Can you work these out from the drawing? Everything is in mm from the part's minimum corner. Give positions to 0.01 mm unless a question says otherwise; leave off trailing zeros. Order: outer loops, then holes, each group sorted by start corner. A loop starts at its lowest first (then second) coordinate and runs counter-clockwise, first axis right, second up. Notation, with made-up numbers: M 2.25,45.5 L 53.25,45.5 A7 ccw 53.25,56.5 Z; hole C 26,11 d3. An arc over 180 degrees is marked long. Answer as a JSON object with one key per item and string values.
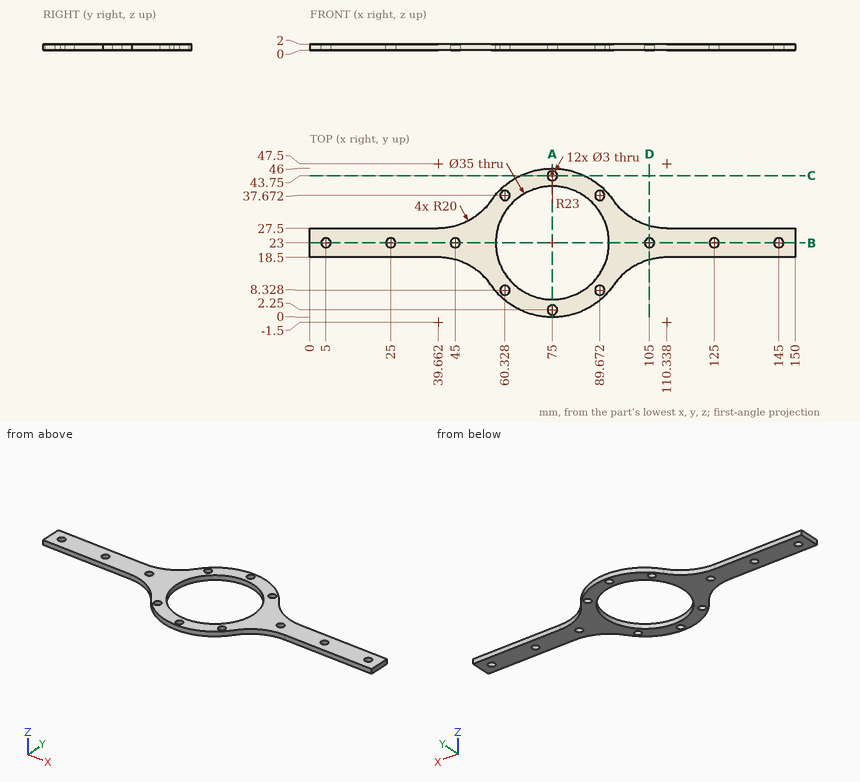
1) I want a section at A-A on x = 75. Write out the boundary of the cut face in (y, z).
Results found:
{"outline": "M 0,0 L 0.75,0 L 0.75,2 L 0,2 Z; M 3.75,0 L 5.5,0 L 5.5,2 L 3.75,2 Z; M 40.5,0 L 42.25,0 L 42.25,2 L 40.5,2 Z; M 45.25,0 L 46,0 L 46,2 L 45.25,2 Z"}
2) I'm going to push flat-ended pins straight in: pin 1 Ø1.8 at (x, y) = (145, 23) entering from +Z; pin 2 Ø1 at (y, z) = (11.5, 1.5) entering from +X; pin 3 Ø3.5 at (x, y) = (45, 23) entering from +Z; pin 4 Ø1 at (x, z) = (131.5, 0.5) entering from -Y. Where does each tip first touch, or does it pass through?
Results found:
{"pin 1": "passes through", "pin 2": "stops at x = 95.58", "pin 3": "stops at z = 2", "pin 4": "stops at y = 18.5"}
3) I need wall thicknesses on L1, parallel to Y at x = 75, z = 0.5; L2, parallel to X at y = 33.5, z = 0.4 (1 decimal); L3, parallel to Y at x = 105, z = 0.9 (1 decimal). Which ranges of each line are inside material? Lowest first, please.
Results found:
{"L1": "y = 0 to 0.75, 3.75 to 5.5, 40.5 to 42.25, 45.25 to 46", "L2": "x = 53.9 to 61, 89 to 96.1", "L3": "y = 17.8 to 21.5, 24.5 to 28.2"}
4) I want a section at D-D on x = 105. Write out the boundary of the cut face in (y, z) (1 decimal).
Results found:
{"outline": "M 17.8,0 L 21.5,0 L 21.5,2 L 17.8,2 Z; M 24.5,0 L 28.2,0 L 28.2,2 L 24.5,2 Z"}
5) I want a section at B-B on y = 23. Count the separate pieces of the cut face and the enclosed holes in it, and give its area (3 significant figures).
Results found:
{"separate pieces": "8", "enclosed holes": "0", "area": "194 mm²"}
6) I want a section at C-C on y = 43.75. Write out the boundary of the cut face in (x, z).
Results found:
{"outline": "M 65.08,0 L 73.5,0 L 73.5,2 L 65.08,2 Z; M 76.5,0 L 84.92,0 L 84.92,2 L 76.5,2 Z"}
